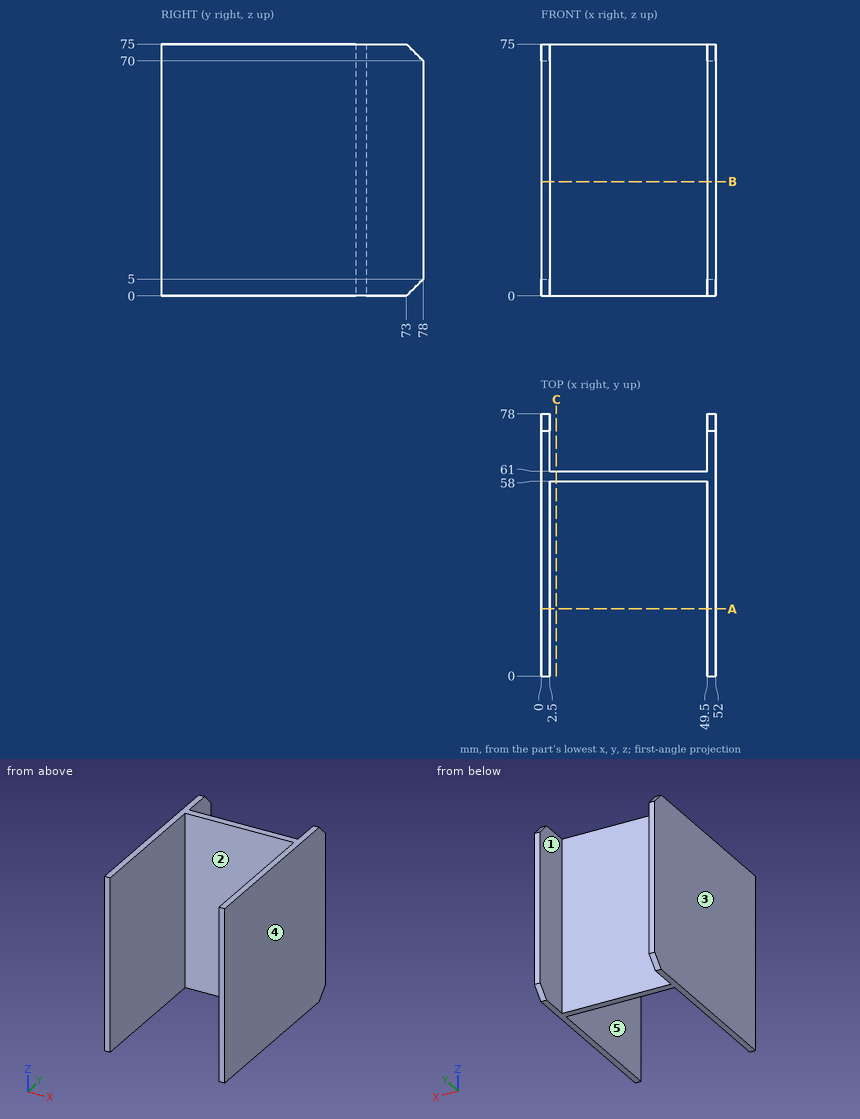
Here's the drawing with two shaded views (mm, measured from the low corner). I have some questions. A direction names the side the tool comes from. Round coordinates to 2 decimals unless told otherwise and drop trailing zeros. Order: outer loops, then holes, each group sorted by start corner. A loop starts at its lowest first (then second) coordinate and runs counter-clockwise, first axis right, second up. Notation, with made-up numbers: (15, 73) -> (20, 73) arc R24 cw to (20, 97) -> close; hole circle Ø7 at (-18.5, 69.5). An arc over 180 degrees is marked (long way). Use a Markdown table: item, result. Add a question column.
(1) Suppose I cut it at C-C, the plane x = 4.5. Please give me the cut outline in (y, z), and give its area (3 significant figures).
(2) For the marked faces 1 and 2, which set-ups out of +Z, -Z, +X, -X, +Y, -Y let a thin tool reach every point of the face, with its end or its side?
(3) Suppose I cut it at B-B, the plane z = 34. Please give me the cut outline in (x, y).
(4) Suppose I cut it at A-A, the plane y = 20. Please give me the cut outline in (x, z).
(5) I need wall thicknesses on line 1 along X through (y, z) = (54, 50); line 2 along Y through (x, z) = (23, 11). Which ranges of each line are inside material? Lowest first, please.
(6) For pin 1 Ø4 at (x, z) = (20.5, 35.5) entering from +Y, with a flat end and sliding along its axis, tell me the tip position at first contact or that it passes through.
(7) If we mould it in two halves opening along X, with no side actions, what happens to the marked faces 3, 4 and 5? For each: released by +X, released by -X, zero draft, split by the parting line, or undercut.
Verdict:
| question | item | result |
|---|---|---|
| 1 | outline | (58, 0) -> (61, 0) -> (61, 75) -> (58, 75) -> close |
| 1 | area | 225 mm2 |
| 2 | face 1 | +Z, -Z, +Y |
| 2 | face 2 | +Z, -Z, -Y |
| 3 | outline | (0, 0) -> (2.5, 0) -> (2.5, 58) -> (49.5, 58) -> (49.5, 0) -> (52, 0) -> (52, 78) -> (49.5, 78) -> (49.5, 61) -> (2.5, 61) -> (2.5, 78) -> (0, 78) -> close |
| 4 | outline | (0, 0) -> (2.5, 0) -> (2.5, 75) -> (0, 75) -> close; (49.5, 0) -> (52, 0) -> (52, 75) -> (49.5, 75) -> close |
| 5 | line 1 | 0 to 2.5, 49.5 to 52 |
| 5 | line 2 | 58 to 61 |
| 6 | pin 1 | y = 61 |
| 7 | face 3 | released by -X |
| 7 | face 4 | released by +X |
| 7 | face 5 | undercut |
